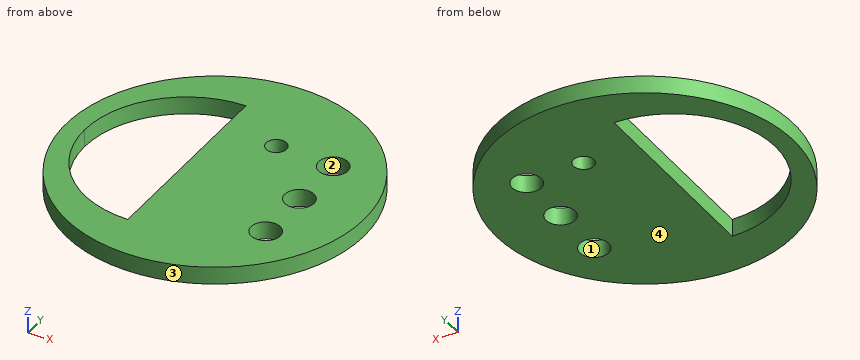
from build123d import *

# Parameters (mm, degrees)
F0_R     = 51
F0_R_2   = 5
F0_R_3   = 3.5
F1_DEPTH = 6


with BuildPart() as f1:
    # F0 (on Top) → F1 (new body)
    with BuildSketch(Plane.XY):
        Circle(F0_R)
        with Locations((28.914182, -20)):
            Circle(F0_R_2, mode=Mode.SUBTRACT)
        with BuildLine():
            ThreePointArc((-44.63806, 0), (-34.386797, 24.748737), (-9.63806, 35))
            Line((-9.63806, 35), (-9.63806, -35))
            ThreePointArc((-9.63806, -35), (-34.386797, -24.748737), (-44.63806, 0))
        make_face(mode=Mode.SUBTRACT)
        with Locations((8.914182, 20.921642)):
            Circle(F0_R_3, mode=Mode.SUBTRACT)
        with Locations((28.914182, 0)):
            Circle(F0_R_2, mode=Mode.SUBTRACT)
        with Locations((28.914182, 20)):
            Circle(F0_R_2, mode=Mode.SUBTRACT)
    extrude(amount=F1_DEPTH)


solid = f1.part
Geometry check sheet. Reference: the model listing, model coordinates, mm. Face numbers are marked on the shaded views. Coordinates: 2 decimals unless noted, no trailing zeros. Order: outer loops, then holes, each group sorted by start corner. A loop starts at its lowest first (then second) coordinate and runs counter-clockwise, first axis right, second up. Notation, with made-up numbers: (48.25, 84.25) -> (65.25, 84.25) arc R15 cw to (65.25, 95.25) -> close; hole circle Ø10 at (-24.5, 18.25). An arc over 180 degrees is marked (long way). Use a Markdown table: item, result. Add a question column.
1. Cross-section at A-A (y = -27). Enter the section's corners in (x, z).
2. Material ranges on L1, parallel to X at y = -2, z = 0.75; L2, parallel to X at y = -23.5, z = 1.7; L3, parallel to Y at x = -34.5, z = 3.1, recorded low to high.
3. Cross-section at D-D (y = 28.5). Enter the section's corners in (x, z), and give its area (3 significant figures).
4. Cross-section at C-C (x = 28). Enter the section's corners in (y, z), and give its area (3 significant figures).
5. Go/stop test with flat-tipped pins: pin 1 Ø1 at (x, z) = (-24, 1.5) entering from -Y; pin 2 Ø16 at (x, y) = (28.91, 0) entering from +Z. Record where each tip stops, or that it passes through.
6. Mould release check, pull along X, two halves, no side actions. Record for the marked faces 1, 2, 3 and 4: pulls with the +X half, pulls with the -X half, needs draft (parallel to the pull), parting line crosses it, or undercut.
7. Cross-section at B-B (z = 3.4). Enter the section's corners in (x, y).
Filled sheet:
| question | item | result |
|---|---|---|
| 1 | outline | (-43.27, 0) -> (-31.91, 0) -> (-31.91, 6) -> (-43.27, 6) -> close; (-9.64, 0) -> (43.27, 0) -> (43.27, 6) -> (-9.64, 6) -> close |
| 2 | L1 | -50.96 to -44.58, -9.64 to 24.33, 33.5 to 50.96 |
| 2 | L2 | -45.26 to -35.58, -9.64 to 25.34, 32.48 to 45.26 |
| 2 | L3 | -37.56 to -24.64, 24.64 to 37.56 |
| 3 | outline | (-42.29, 0) -> (-29.95, 0) -> (-29.95, 6) -> (-42.29, 6) -> close; (-9.64, 0) -> (42.29, 0) -> (42.29, 6) -> (-9.64, 6) -> close |
| 3 | area | 386 mm2 |
| 4 | outline | (-42.63, 0) -> (-24.92, 0) -> (-24.92, 6) -> (-42.63, 6) -> close; (-15.08, 0) -> (-4.92, 0) -> (-4.92, 6) -> (-15.08, 6) -> close; (4.92, 0) -> (15.08, 0) -> (15.08, 6) -> (4.92, 6) -> close; (24.92, 0) -> (42.63, 0) -> (42.63, 6) -> (24.92, 6) -> close |
| 4 | area | 335 mm2 |
| 5 | pin 1 | y = -45.26 |
| 5 | pin 2 | z = 6 |
| 6 | face 1 | undercut |
| 6 | face 2 | undercut |
| 6 | face 3 | parting line crosses it |
| 6 | face 4 | needs draft |
| 7 | outline | circle Ø102 at (0, 0); hole (-44.64, 0) arc R35 ccw to (-9.64, -35) -> (-9.64, 35) arc R35 ccw to start; hole circle Ø7 at (8.91, 20.92); hole circle Ø10 at (28.91, -20); hole circle Ø10 at (28.91, 0); hole circle Ø10 at (28.91, 20) |
